Geometry: final body of the model. Coordinates: model frame, mm. Round coordinates to 2 decimals unless told otherwise and drop trailing zeros. Loops run counter-clockwise (first coordinate to the right, second up) from the corner with the lowest first, then second, coordinate; pieces in that order, holes last. Notation, with made-up numbers: (-21, 62) - (-1, 62) arc R29 ccw to (-1, 95) - close; hole circle Ø5 at (10.25, 25.25). An arc over 180 degrees is marked (long way). Write item = value, one per line. Start each with the question number.
Item 1: Section B-B (x = -12.7). Return loops of the section in (y, z), plus the area to 3 significant figures.
Item 2: First-contact query: pin 1 (8 mm diameter, centred on x = 38, y = 28.5, fed in from +Z); pin 2 (7 mm diameter, centred on x = 38, y = -28.5, fed in from -Z). Flat tips, straight axial feed; report the tip coordinate or a pass-through.
Item 3: Line query: line 1 (Y direction, x = -38, z = 7.15); line 2 (Y direction, x = -12.7, z = 6.25); line 3 (Y direction, x = 38, z = 2.45). Output: solid intervals per line, ascending. Write a range as from..to.
Item 4: Section A-A (z = 3.75). Count the separate pieces of the cut face and the enclosed holes in it, plus the area to 3 significant figures.
from build123d import *

# Parameters (mm, degrees)
SKETCH_1_W          = 100
SKETCH_1_H          = 87
EXTRUDE_1_DEPTH     = 10
FILLET_1_R          = 10
SKETCH_2_R          = 2.6
CUT_EXTRUDE_1_DEPTH = 10
SKETCH_3_R          = 5
CUT_EXTRUDE_2_DEPTH = 5
SKETCH_4_R          = 3.1
CUT_EXTRUDE_3_DEPTH = 5
CHAMFER_1_SIZE      = 1
CHAMFER_2_SIZE      = 2


with BuildPart() as part:
    # 草图1 → 凸台-拉伸1 (new body)
    with BuildSketch(Plane.XY):
        Rectangle(SKETCH_1_W, SKETCH_1_H)
    extrude(amount=EXTRUDE_1_DEPTH)

    # 圆角1
    fillet_1_edges = [part.edges().sort_by_distance(p)[0] for p in [
        (50, -43.5, 5),
        (-50, -43.5, 5),
        (-50, 43.5, 5),
        (50, 43.5, 5),
    ]]
    fillet(fillet_1_edges, radius=FILLET_1_R)

    # 草图2 → 切除-拉伸1 (cut)
    with BuildSketch(Plane.XY.offset(10)):
        with Locations((0, 32)):
            Circle(SKETCH_2_R)
        with Locations((-12.7, 32)):
            Circle(SKETCH_2_R)
        with Locations(Location((12.7, 32, 0), (0, 0, 180))):
            Circle(SKETCH_2_R)
        with Locations((-12.7, -32)):
            Circle(SKETCH_2_R)
        with Locations((0, -32)):
            Circle(SKETCH_2_R)
        with Locations((12.7, -32)):
            Circle(SKETCH_2_R)
    extrude(amount=-CUT_EXTRUDE_1_DEPTH, mode=Mode.SUBTRACT)

    # 草图3 → 切除-拉伸2 (cut)
    with BuildSketch(Plane.XY.offset(10)):
        with Locations((-38, 28.5)):
            Circle(SKETCH_3_R)
        with Locations((-38, 0)):
            Circle(SKETCH_3_R)
        with Locations((-38, -28.5)):
            Circle(SKETCH_3_R)
        with Locations(Location((38, -28.5, 0), (0, 0, 180))):
            Circle(SKETCH_3_R)
        with Locations(Location((38, 0, 0), (0, 0, 180))):
            Circle(SKETCH_3_R)
        with Locations(Location((38, 28.5, 0), (0, 0, 180))):
            Circle(SKETCH_3_R)
    extrude(amount=-CUT_EXTRUDE_2_DEPTH, mode=Mode.SUBTRACT)

    # 草图4 → 切除-拉伸3 (cut)
    with BuildSketch(Plane.XY.offset(5)):
        with Locations((-38, 28.5)):
            Circle(SKETCH_4_R)
        with Locations((-38, 0)):
            Circle(SKETCH_4_R)
        with Locations((-38, -28.5)):
            Circle(SKETCH_4_R)
        with Locations((38, 28.5)):
            Circle(SKETCH_4_R)
        with Locations((38, 0)):
            Circle(SKETCH_4_R)
        with Locations((38, -28.5)):
            Circle(SKETCH_4_R)
    extrude(amount=-CUT_EXTRUDE_3_DEPTH, mode=Mode.SUBTRACT)

    # 倒角1
    chamfer_1_edges = [part.edges().sort_by_distance(p)[0] for p in [
        (34.9, 0, 0),
        (34.9, -28.5, 0),
        (-41.1, 28.5, 0),
        (-41.1, 0, 0),
        (-41.1, -28.5, 0),
        (34.9, 28.5, 0),
    ]]
    chamfer(chamfer_1_edges, length=CHAMFER_1_SIZE)

    # 倒角2
    chamfer_2_edges = [part.edges().sort_by_distance(p)[0] for p in [
        (0, 43.5, 10),
        (50, 0, 10),
        (-50, 0, 10),
        (0, -43.5, 10),
        (-47.071067812, -40.571067812, 10),
        (47.071067812, -40.571067812, 10),
        (-47.071067812, 40.571067812, 10),
        (47.071067812, 40.571067812, 10),
    ]]
    chamfer(chamfer_2_edges, length=CHAMFER_2_SIZE)


solid = part.part
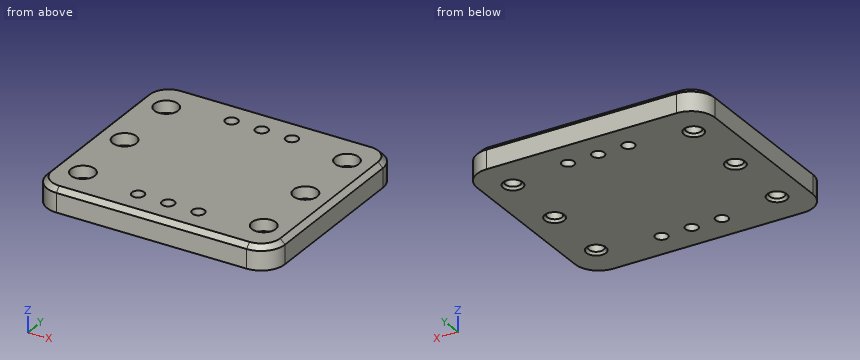
Taken from the geometry:
q1.outline = (-43.5, 0) - (-34.6, 0) - (-34.6, 10) - (-41.5, 10) - (-43.5, 8) - close; (-29.4, 0) - (29.4, 0) - (29.4, 10) - (-29.4, 10) - close; (34.6, 0) - (43.5, 0) - (43.5, 8) - (41.5, 10) - (34.6, 10) - close
q1.area = 762 mm^2
q2.pin_1 = 5
q2.pin_2 = 0.6
q3.line_1 = -43.5..-33.5, -23.5..-5, 5..23.5, 33.5..43.5
q3.line_2 = -43.5..-34.6, -29.4..29.4, 34.6..43.5
q3.line_3 = -43.5..-31.6, -25.4..-3.1, 3.1..25.4, 31.6..43.5
q4.separate_pieces = 1
q4.enclosed_holes = 12
q4.area = 8,310 mm^2
